from build123d import *

# Parameters (mm, degrees)
F0_R     = 2
F1_DEPTH = 25
F3_DEPTH = 29.5


with BuildPart() as f1:
    # F0 (on Top) → F1 (new body)
    with BuildSketch(Plane.XY):
        with BuildLine():
            ThreePointArc((2.993309, 22.271687), (0, 25.471937), (-2.993309, 22.271687))
            ThreePointArc((-2.993309, 22.271687), (0, -22.471937), (2.993309, 22.271687))
        make_face()
        with BuildLine():
            Line((-4.766043, -16.90091), (0, -5.909285))
            Line((0, -5.909285), (4.766043, -16.90091))
            ThreePointArc((4.766043, -16.90091), (2.405704, -17.394496), (0, -17.560066))
            ThreePointArc((0, -17.560066), (-2.405704, -17.394496), (-4.766043, -16.90091))
        make_face(mode=Mode.SUBTRACT)
        with BuildLine():
            ThreePointArc((-7.413827, -15.918262), (-15.996416, -7.243657), (-16.854101, 4.929016))
            Line((-16.854101, 4.929016), (-7.413827, -15.918262))
        make_face(mode=Mode.SUBTRACT)
        with BuildLine():
            Line((7.413827, -15.918262), (16.854101, 4.929016))
            ThreePointArc((16.854101, 4.929016), (15.996416, -7.243657), (7.413827, -15.918262))
        make_face(mode=Mode.SUBTRACT)
        with BuildLine():
            ThreePointArc((-14.089574, 10.480449), (-11.809122, 12.996175), (-9.08713, 15.025977))
            Line((-9.08713, 15.025977), (-2.853133, 0.640048))
            Line((-2.853133, 0.640048), (0, 0.640048))
            Line((0, 0.640048), (2.853133, 0.640048))
            Line((2.853133, 0.640048), (9.08713, 15.025977))
            ThreePointArc((9.08713, 15.025977), (11.809122, 12.996175), (14.089574, 10.480449))
            Line((14.089574, 10.480449), (5.919134, -7.606121))
            Line((5.919134, -7.606121), (2.806974, -0.579698))
            Line((2.806974, -0.579698), (0, -0.579698))
            Line((0, -0.579698), (-2.806974, -0.579698))
            Line((-2.806974, -0.579698), (-5.919134, -7.606121))
            Line((-5.919134, -7.606121), (-14.089574, 10.480449))
        make_face(mode=Mode.SUBTRACT)
        with BuildLine():
            Line((0, 5.937309), (-4.799841, 16.891342))
            ThreePointArc((-4.799841, 16.891342), (-2.423101, 17.392081), (0, 17.560066))
            ThreePointArc((0, 17.560066), (2.423101, 17.392081), (4.799841, 16.891342))
            Line((4.799841, 16.891342), (0, 5.937309))
        make_face(mode=Mode.SUBTRACT)
        with Locations((0, 22.471937)):
            Circle(F0_R, mode=Mode.SUBTRACT)
    extrude(amount=F1_DEPTH)

    # F2 (on Front) → F3 (cut, symmetric)
    with BuildSketch(Plane.XZ):
        with BuildLine():
            ThreePointArc((-25, 14.797118), (0, 22.984089), (25, 14.797118))
            Line((25, 14.797118), (25.056494, 26.376059))
            Line((25.056494, 26.376059), (-25, 26.376059))
            Line((-25, 26.376059), (-25, 14.797118))
        make_face()
    extrude(amount=F3_DEPTH, both=True, mode=Mode.SUBTRACT)


solid = f1.part
Check sheet for the modelled part. Datum: model origin and axes. Units: mm. A direction names the side the tool comes from. Round coordinates to 2 decimals unless told otherwise and drop trailing zeros. Loops run counter-clockwise (first coordinate to the right, second up) from the corner with the lowest first, then second, coordinate; pieces in that order, holes last. Notation, with made-up numbers: (4, 74.25) -> (14, 74.25) arc R22 ccw to (14, 98.25) -> close; hole circle Ø4 at (29.5, 18). An arc over 180 degrees is marked (long way). Put each result on its own line as item: value. Start each with the question number.
1. Section check A-A (y = 12). Enter the section's corners in (x, z), plus the area to 3 significant figures.
2. Section check C-C (z = 9.75). Enter the section's corners in (x, y), plus the area to 3 significant figures.
3. Gauge pin test, flat ends, axial feed: pin 1 (5 mm diameter, centred on x = -2.5, y = 3.5, fed in from +Z); pin 2 (3 mm diameter, centred on x = 2.5, z = 7.5, fed in from +Y); pin 3 (5 mm diameter, centred on y = -12.5, z = 20, fed in from +X); pin 4 (4 mm diameter, centred on y = 16, z = 19, fed in from +X). Record the tip position at first contact, or that the pin passes through.
4. Scan lines: probe 1 along Y at (x, z) = (-13, 13.25); probe 2 along X at (y, z) = (2.5, 17); probe 3 along X at (y, z) = (-2, 2.75). Record each from-to range of solid material in increasing order.
5. Section check B-B (y = -7). Enter the section's corners in (x, z), plus the area to 3 significant figures.
6. Access from +Z, -Z, +X, -X, +Y, -Y to the whole of each face (thin tool, end or side, straight path). Record for faces 4 (the face through (-0.332, -4.154, 22.983)), 5 (the face through (0, -0.58, 11)).
7. Draft check along X on faces 1 (the face through (0, -3, 0)), 2 (the face through (-15.924, -7.402, 11.008)), 3 (the face through (0.07, 25.47, 11.33)). Enter one of: +X half, -X half, draft (parallel to the pull), parting line (faces both ways), or undercut.
8. Section check D-D (x = 15). Enter the section's corners in (y, z).
Findings:
1. outline: (-19, 0) -> (-12.82, 0) -> (-12.82, 20.99) arc R42.26 ccw to (-19, 18.47) -> close; (-7.78, 0) -> (-2.66, 0) -> (-2.66, 22.9) arc R42.26 ccw to (-7.78, 22.26) -> close; (2.66, 0) -> (7.78, 0) -> (7.78, 22.26) arc R42.26 ccw to (2.66, 22.9) -> close; (12.82, 0) -> (19, 0) -> (19, 18.47) arc R42.26 ccw to (12.82, 20.99) -> close
1. area: 477 mm^2
2. outline: (-2.99, 22.27) arc R22.47 ccw (long way) to (2.99, 22.27) arc R3 ccw (long way) to start; hole (-16.85, 4.93) arc R17.56 ccw to (-7.41, -15.92) -> close; hole (-14.09, 10.48) -> (-5.92, -7.61) -> (-2.81, -0.58) -> (2.81, -0.58) -> (5.92, -7.61) -> (14.09, 10.48) arc R17.56 ccw to (9.09, 15.03) -> (2.85, 0.64) -> (-2.85, 0.64) -> (-9.09, 15.03) arc R17.56 ccw to start; hole (-4.8, 16.89) -> (0, 5.94) -> (4.8, 16.89) arc R17.56 ccw to (0, 17.56) arc R17.56 ccw to start; hole (-4.77, -16.9) arc R17.56 ccw to (0, -17.56) arc R17.56 ccw to (4.77, -16.9) -> (0, -5.91) -> close; hole circle Ø4 at (0, 22.47); hole (7.41, -15.92) arc R17.56 ccw to (16.85, 4.93) -> close
2. area: 1,100 mm^2
3. pin 1: stops at z = 22.98
3. pin 2: stops at y = 25.3
3. pin 3: stops at x = 19.68
3. pin 4: stops at x = 17.58
4. probe 1: y = -18.33 to -11.8, -3.58 to 8.07, 11.8 to 18.33
4. probe 2: x = -21.68 to -17.38, -15.75 to -10.48, -3.66 to 3.66, 10.48 to 15.75, 17.38 to 21.68
4. probe 3: x = -22.38 to -17.45, -13.72 to -8.45, -3.44 to 3.44, 8.45 to 13.72, 17.45 to 22.38
5. outline: (-21.35, 0) -> (-16.1, 0) -> (-16.1, 19.8) arc R42.26 ccw to (-21.35, 17.19) -> close; (-11.45, 0) -> (-6.19, 0) -> (-6.19, 22.53) arc R42.26 ccw to (-11.45, 21.4) -> close; (-5.65, 0) -> (-0.47, 0) -> (-0.47, 22.98) arc R42.26 ccw to (-5.65, 22.6) -> close; (0.47, 0) -> (5.65, 0) -> (5.65, 22.6) arc R42.26 ccw to (0.47, 22.98) -> close; (6.19, 0) -> (11.45, 0) -> (11.45, 21.4) arc R42.26 ccw to (6.19, 22.53) -> close; (16.1, 0) -> (21.35, 0) -> (21.35, 17.19) arc R42.26 ccw to (16.1, 19.8) -> close
5. area: 663 mm^2
6. face 4: +Z, +Y, -Y
6. face 5: +Z, -Z
7. face 1: draft
7. face 2: undercut
7. face 3: parting line
8. outline: (-16.73, 0) -> (-9.13, 0) -> (-9.13, 20.23) -> (-16.73, 20.23) -> close; (0.83, 0) -> (16.73, 0) -> (16.73, 20.23) -> (0.83, 20.23) -> close
